Here's the drawing with two shaded views (mm, measured from the low corner). I have some questions. Round coordinates to 2 decimals unless told otherwise and drop trailing zeros. Order: outer loops, then holes, each group sorted by start corner. A loop starts at its lowest first (then second) coordinate and runs counter-clockwise, first axis right, second up. Notation, with made-up numbers: M 16.5,29 L 69.5,29 A17 cw 69.5,51 Z; hole C -4.5,76.25 d6. An arc over 180 degrees is marked long. One line per question, with ' | ' between items.
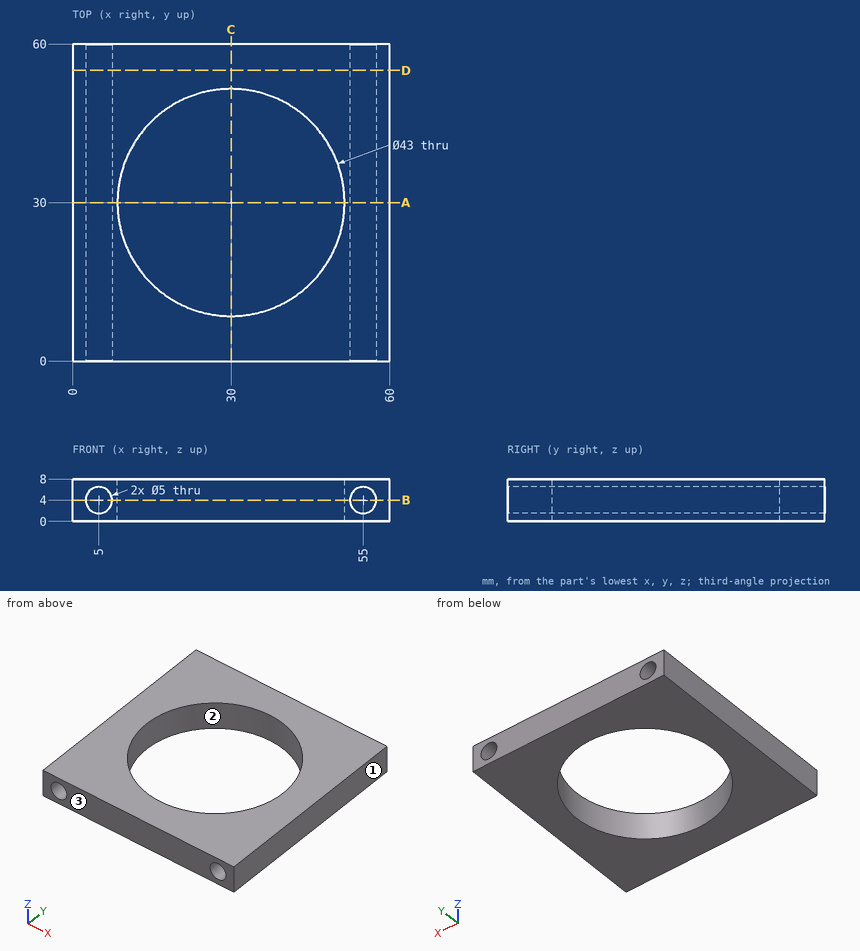
(1) If we section it at C-C on x = 30: Please give me the cut outline in (y, z).
Final values:
outline: M 0,0 L 8.5,0 L 8.5,8 L 0,8 Z; M 51.5,0 L 60,0 L 60,8 L 51.5,8 Z
(2) Please list where these lines run through material, in increasing order: probe 1 along Z at (x, y) = (55, 42); probe 2 along Y at (x, z) = (30, 2.25); probe 3 along X at (y, z) = (41, 4.5). Write a range as [from, to].
Final values:
probe 1: [0, 1.5], [6.5, 8] | probe 2: [0, 8.5], [51.5, 60] | probe 3: [0, 2.55], [7.45, 11.53], [48.47, 52.55], [57.45, 60]
(3) Will these pins go through, and if not, where does the flat tip stop? pin 1 Ø12 at (x, y) = (30.5, 15.5) entering from +Z; pin 2 Ø1.5 at (x, y) = (48.5, 43) entering from -Z.
Final values:
pin 1: through | pin 2: z = 0
(4) If we section it at D-D on y = 55: Please give me the cut outline in (x, z).
Final values:
outline: M 0,0 L 60,0 L 60,8 L 0,8 Z; hole C 5,4 d5; hole C 55,4 d5
(5) If we section it at B-B on z = 4: Please give me the cut outline in (x, y).
Final values:
outline: M 0,0 L 2.5,0 L 2.5,60 L 0,60 Z; M 7.5,0 L 52.5,0 L 52.5,60 L 7.5,60 Z; M 57.5,0 L 60,0 L 60,60 L 57.5,60 Z; hole C 30,30 d43
(6) If we section it at A-A on y = 30: Please give me the cut outline in (x, z), plus the area to 3 significant figures.
Final values:
outline: M 0,0 L 8.5,0 L 8.5,8 L 0,8 Z; M 51.5,0 L 60,0 L 60,8 L 51.5,8 Z; hole C 5,4 d5; hole C 55,4 d5 | area: 96.7 mm^2
(7) Thinking about a two-plate mould opening in Y: for the marked faces 1, 2 and 3, which applies, released by +Y, released by -Y, zero draft, split by the parting line, or undercut?
Final values:
face 1: zero draft | face 2: undercut | face 3: released by -Y
